For this review, take the finished solid that the model builds, in its own axes (mm). A direction names the side the tool comes from. Give positions to 0.01 mm unless a question says otherwise; leave off trailing zeros. Loops run counter-clockwise (first coordinate to the right, second up) from the corner with the lowest first, then second, coordinate; pieces in that order, holes last. Notation, with made-up numbers: (1, 76) - (20, 76) arc R6 cw to (20, 82) - close; hole circle Ø10 at (63.5, 7). An arc over 180 degrees is marked (long way). Use CSV: the item, a comma, the result in double quotes. Start each with the question number.
1. For faces 1 (the flat face through (0, -2, 16)), 2 (the flat face through (-19.5, -2, 0)), 3 (the flat face through (0, -2, -16)), 4 (the flat face through (19.5, -2, 0)), list the 3-axis set-ups (+Z, -Z, +X, -X, +Y, -Y) from which the entire face can be reached by the end or side of a thin tool; tool diameter is ignored.
2. Wall thickness on line 1 (X direction, y = -2.35, z = 15); line 2 (Z direction, x = 12, y = -1.55); line 3 (Y direction, x = -22.5, z = 10.5): over which ranges is each line inside the solid? List them lowest first.
3. Take a section at C-C on y = -0.9. Give the boundary of the cut face in (x, z).
4. For pin 1 (3 mm diameter, centred on x = -23, z = -11, fed in from +Y); pin 2 (1.5 mm diameter, centred on y = -2.5, z = 12, fed in from +X); pin 3 (2.5 mm diameter, centred on y = -1, z = -6, fed in from +X); pin 4 (0.9 mm diameter, centred on x = 9, y = -2, fed in from -Z), all flat-tipped, find the tip position at first contact; note any pin that passes through.
5. Take a section at D-D on x = 22. Give the boundary of the cut face in (y, z).
6. Take a section at B-B on x = 14. Give the boundary of the cut face in (y, z).
7. Take a section at A-A on z = -3. Give the boundary of the cut face in (x, y), plus the area to 3 significant figures.
```python
from build123d import *

# Parameters (mm, degrees)
LCD_GLASS_START = -3
SKETCH1_W       = 39
SKETCH1_H       = 32
LCD_GLASS_DEPTH = 3
BOARD_START     = -4.6
SKETCH2_W       = 58
SKETCH2_H       = 35
BOARD_DEPTH     = 1.6


with BuildPart() as part:
    # Sketch1 → LCD_Glass (new body)
    with BuildSketch(Plane(origin=(0, 0, 0), x_dir=(1, 0, 0), z_dir=(0, 1, 0)).offset(LCD_GLASS_START)):
        Rectangle(SKETCH1_W, SKETCH1_H)
    extrude(amount=LCD_GLASS_DEPTH)

    # Sketch2 → Board (add)
    with BuildSketch(Plane(origin=(0, 0, 0), x_dir=(1, 0, 0), z_dir=(0, 1, 0)).offset(BOARD_START)):
        Rectangle(SKETCH2_W, SKETCH2_H)
    extrude(amount=BOARD_DEPTH)


solid = part.part
```
Check result:
1,face 1,"+Z, +X, -X, +Y"
1,face 2,"+Z, -Z, -X, +Y"
1,face 3,"-Z, +X, -X, +Y"
1,face 4,"+Z, -Z, +X, +Y"
2,line 1,"x = -19.5 to 19.5"
2,line 2,"z = -16 to 16"
2,line 3,"y = -4.6 to -3"
3,outline,"(-19.5, -16) - (19.5, -16) - (19.5, 16) - (-19.5, 16) - close"
4,pin 1,"stops at y = -3"
4,pin 2,"stops at x = 29"
4,pin 3,"stops at x = 19.5"
4,pin 4,"stops at z = -16"
5,outline,"(-4.6, -17.5) - (-3, -17.5) - (-3, 17.5) - (-4.6, 17.5) - close"
6,outline,"(-4.6, -17.5) - (-3, -17.5) - (-3, -16) - (0, -16) - (0, 16) - (-3, 16) - (-3, 17.5) - (-4.6, 17.5) - close"
7,outline,"(-29, -4.6) - (29, -4.6) - (29, -3) - (19.5, -3) - (19.5, 0) - (-19.5, 0) - (-19.5, -3) - (-29, -3) - close"
7,area,"210 mm²"
